Geometry check sheet. Reference: the model listing, model coordinates, mm. Face numbers are marked on the shaded views. Coordinates: 2 decimals unless noted, no trailing zeros. Write each loop counter-clockwise with the first axis right and the second up, starting at its lowest first coordinate (ties: lowest second). Pieces come first, ordered by that corner, then holes. Notation, with made-up numbers: (26.25, 24) -> (79.25, 24) arc R4 ccw to (79.25, 29) -> close; hole circle Ø4 at (-39, 18.5). An arc over 180 degrees is marked (long way). One line per question, with ' | ' between items.
```python
from build123d import *

# Parameters (mm, degrees)
F1_DEPTH = 97.5
F3_DEPTH = 28
F4_R     = 4.25
F5_DEPTH = 25
F6_R     = 5.25
F7_DEPTH = 25
F8_R     = 5.25
F9_DEPTH = 25
F10_R    = 2
F11_R    = 0.5
F12_R    = 1


# Not quite as in the source:
# - a pattern or mirror of a feature is missing from the dataset's text; its kind, count and spacing are read off the source's solid


with BuildPart() as f1:
    # F0 (on Top) → F1 (new body, symmetric)
    with BuildSketch(Plane.XY):
        Polygon((-19.75, 3.25), (-19.75, -19.75), (-9.25, -19.75), (19.75, 9.25), (19.75, 19.75), (-3.25, 19.75), (-3.25, 16.75), (16.75, 16.75), (16.75, 10.4926406871), (-10.4926406871, -16.75), (-16.75, -16.75), (-16.75, 3.25), align=None)
    extrude(amount=F1_DEPTH, both=True)

    # F2 (on face) → F3 (cut)
    with BuildSketch(Plane.XY.offset(97.5)):
        Polygon((-10.4926406871, -16.75), (-16.75, -16.75), (-19.75, -16.75), (-19.75, -19.75), (-9.25, -19.75), (19.75, 9.25), (19.75, 19.75), (16.75, 19.75), (16.75, 16.75), (16.75, 10.4926406871), align=None)
    f3 = extrude(amount=-F3_DEPTH, mode=Mode.SUBTRACT)

    # F3_copies: F3 across plane
    add(f3.mirror(Plane(origin=(0, 0, 0), x_dir=(-1, 0, 0), z_dir=(0, 0, -1))), mode=Mode.SUBTRACT)

    # F4 (on face) → F5 (cut)
    with BuildSketch(Plane(origin=(5.25, -5.25, 0), x_dir=(0.7071067812, 0.7071067812, 0), z_dir=(0.7071067812, -0.7071067812, 0))):
        with Locations((0, 42)):
            Circle(F4_R)
        with Locations((0, -42)):
            Circle(F4_R)
        Circle(F4_R)
    extrude(amount=-F5_DEPTH, mode=Mode.SUBTRACT)

    # F6 (on face) → F7 (cut)
    with BuildSketch(Plane.YZ.offset(-16.75)):
        with Locations((-6.75, 85.5)):
            Circle(F6_R)
        with Locations((-6.75, -85.5)):
            Circle(F6_R)
    extrude(amount=-F7_DEPTH, mode=Mode.SUBTRACT)

    # F8 (on face) → F9 (cut)
    with BuildSketch(Plane.XZ.offset(-16.75)):
        with Locations((6.75, 85.5)):
            Circle(F8_R)
        with Locations((6.75, -85.5)):
            Circle(F8_R)
    extrude(amount=-F9_DEPTH, mode=Mode.SUBTRACT)

    # F10
    f10_edges = [f1.edges().sort_by_distance(p)[0] for p in [
        (-9.25, -19.75, 0),
        (19.75, 9.25, 0),
        (-18.25, -16.75, 97.5),
        (-18.25, 3.25, 97.5),
        (-3.25, 18.25, 97.5),
        (16.75, 18.25, 97.5),
        (-18.25, 3.25, -97.5),
        (-3.25, 18.25, -97.5),
        (-18.25, -16.75, -97.5),
        (16.75, 18.25, -97.5),
    ]]
    fillet(f10_edges, radius=F10_R)

    # F11
    f11_edges = [f1.edges().sort_by_distance(p)[0] for p in [
        (16.75, 10.492641, 0),
        (-10.492641, -16.75, 0),
    ]]
    fillet(f11_edges, radius=F11_R)

    # F12
    f12_edges = [f1.edges().sort_by_distance(p)[0] for p in [
        (-19.75, -19.75, 0),
        (19.75, 19.75, 0),
    ]]
    fillet(f12_edges, radius=F12_R)


solid = f1.part
```
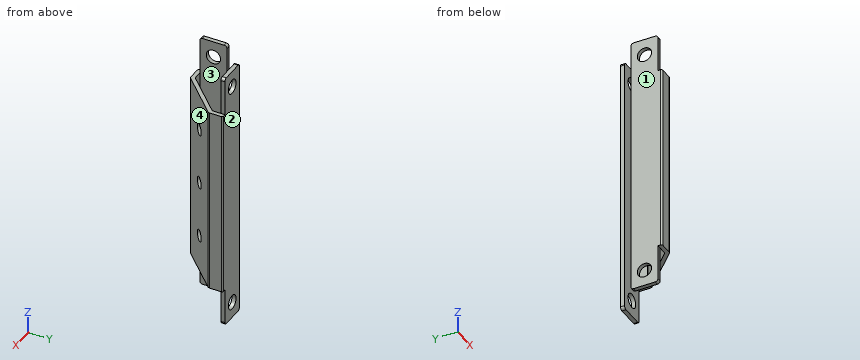
(1) Depth check by flat-ended pin: P1, Ø1.5, axis at x = -17.5, z = 28, coming from the +Y side; P2, Ø1.5, axis at x = -0.5, z = -50.5, coming from the -Y side; P3, Ø3, axis at y = 8.5, z = 16.5, coming from the +X side; P4, Ø1.8, axis at x = -14.5, z = -27.5, coming from the +Y side. Enter the tip coordinate at first touch or a pass-through.
Answers below:
P1: stops at y = 3.25 | P2: stops at y = -11.75 | P3: stops at x = 19.75 | P4: stops at y = -16.75
(2) Cross-section at D-D (x = -12.5). Record the cut outline in (y, z), plus the area to 3 significant figures.
Answers below:
outline: (-19.75, -69.5) -> (-16.75, -69.5) -> (-16.75, 69.5) -> (-19.75, 69.5) -> close | area: 417 mm²
(3) Draft check along X on the marked faces 1, 2, 3 and 4. Enter one of: pulls with the +X half, pulls with the -X half, needs draft (parallel to the pull), parting line crosses it, or undercut.
Answers below:
face 1: pulls with the -X half | face 2: needs draft | face 3: undercut | face 4: pulls with the +X half
(4) Material ranges on line 1 (Z direction, x = -18.95, y = -6.75); line 2 (Y direction, x = 12.5, z = 70.5); line 3 (Z direction, x = 7.5, y = -2.5), recorded low to high.
Answers below:
line 1: z = -97.5 to -90.75, -80.25 to 80.25, 90.75 to 97.5 | line 2: y = 16.75 to 19.75 | line 3: z = -69.5 to -44.36, -39.64 to -2.36, 2.36 to 39.64, 44.36 to 69.5
(5) Cross-section at A-A (z = 85.5). Record the cut outline in (x, y), plus the area to 3 significant figures.
Answers below:
outline: (-19.75, -16.75) -> (-16.75, -16.75) -> (-16.75, -12) -> (-19.75, -12) -> close; (-19.75, -1.5) -> (-16.75, -1.5) -> (-16.75, 3.25) -> (-19.75, 3.25) -> close; (-3.25, 16.75) -> (1.5, 16.75) -> (1.5, 19.75) -> (-3.25, 19.75) -> close; (12, 16.75) -> (16.75, 16.75) -> (16.75, 19.75) -> (12, 19.75) -> close | area: 57.0 mm²
(6) Cross-section at B-B (z = -78). Record the cut outline in (x, y).
Answers below:
outline: (-19.75, -16.75) -> (-16.75, -16.75) -> (-16.75, 3.25) -> (-19.75, 3.25) -> close; (-3.25, 16.75) -> (16.75, 16.75) -> (16.75, 19.75) -> (-3.25, 19.75) -> close
(7) Cross-section at C-C (z = -24). Record the cut outline in (x, y), plus the area to 3 significant figures.
Answers below:
outline: (-19.75, -18.75) arc R1 ccw to (-18.75, -19.75) -> (-10.08, -19.75) arc R2 ccw to (-8.66, -19.16) -> (19.16, 8.66) arc R2 ccw to (19.75, 10.08) -> (19.75, 18.75) arc R1 ccw to (18.75, 19.75) -> (-3.25, 19.75) -> (-3.25, 16.75) -> (16.75, 16.75) -> (16.75, 10.7) arc R0.5 cw to (16.6, 10.35) -> (-10.35, -16.6) arc R0.5 cw to (-10.7, -16.75) -> (-16.75, -16.75) -> (-16.75, 3.25) -> (-19.75, 3.25) -> close | area: 298 mm²
